from build123d import *

# Parameters (mm, degrees)
SKETCH_R        = 1.2
PAD_DEPTH       = 7
SKETCH001_W     = 3.3
SKETCH001_H     = 5
POCKET_DEPTH    = 50
SKETCH002_W     = 3.3
SKETCH002_H     = 5
POCKET001_DEPTH = 30
CHAMFER_SIZE    = 2.5
FILLET_R        = 1
FILLET001_R     = 1


with BuildPart() as part:
    # Sketch → Pad (new body)
    with BuildSketch(Plane.XY):
        Polygon((-4.5, 23), (4.5, 23), (4.5, 4.5), (9.5, 4.5), (9.5, -4.5), (4.5, -4.5), (4.5, -23), (-4.5, -23), (-4.5, -4.5), (-9.5, -4.5), (-9.5, 4.5), (-4.5, 4.5), align=None)
        with Locations((0, 15.5)):
            Circle(SKETCH_R, mode=Mode.SUBTRACT)
        with Locations((0, -15.5)):
            Circle(SKETCH_R, mode=Mode.SUBTRACT)
    extrude(amount=PAD_DEPTH)

    # Sketch001 → Pocket (cut)
    with BuildSketch(Plane(origin=(0, 23, 0), x_dir=(-1, 0, 0), z_dir=(0, 1, 0))):
        with Locations((0, 4.5)):
            Rectangle(SKETCH001_W, SKETCH001_H)
    extrude(amount=-POCKET_DEPTH, mode=Mode.SUBTRACT)

    # Sketch002 → Pocket001 (cut)
    with BuildSketch(Plane(origin=(-9.5, 0, 0), x_dir=(0, -1, 0), z_dir=(-1, 0, 0))):
        with Locations((0, 4.5)):
            Rectangle(SKETCH002_W, SKETCH002_H)
    extrude(amount=-POCKET001_DEPTH, mode=Mode.SUBTRACT)

    # Chamfer
    chamfer_edges = [part.edges().sort_by_distance(p)[0] for p in [
        (-4.5, 13.75, 7),
        (-7, 4.5, 7),
        (4.5, 13.75, 7),
        (7, 4.5, 7),
        (7, -4.5, 7),
        (4.5, -13.75, 7),
        (-4.5, -13.75, 7),
        (-7, -4.5, 7),
    ]]
    chamfer(chamfer_edges, length=CHAMFER_SIZE)

    # Fillet
    fillet_edges = [part.edges().sort_by_distance(p)[0] for p in [
        (-9.5, 1.65, 4.5),
        (-9.5, -1.65, 4.5),
        (-1.65, 23, 4.5),
        (1.65, 23, 4.5),
        (9.5, 1.65, 4.5),
        (9.5, -1.65, 4.5),
        (-1.65, -23, 4.5),
        (1.65, -23, 4.5),
        (1.65, 1.65, 4.5),
        (-1.65, 1.65, 4.5),
        (1.65, -1.65, 4.5),
        (-1.65, -1.65, 4.5),
    ]]
    fillet(fillet_edges, radius=FILLET_R)

    # Fillet001
    fillet001_edges = [part.edges().sort_by_distance(p)[0] for p in [
        (-9.5, -4.5, 2.25),
        (-9.5, 4.5, 2.25),
        (-4.5, 4.5, 2.25),
        (-4.5, 23, 2.25),
        (4.5, 23, 2.25),
        (4.5, 4.5, 2.25),
        (9.5, 4.5, 2.25),
        (9.5, -4.5, 2.25),
        (4.5, -4.5, 2.25),
        (4.5, -23, 2.25),
        (-4.5, -23, 2.25),
        (-4.5, -4.5, 2.25),
    ]]
    fillet(fillet001_edges, radius=FILLET001_R)


solid = part.part
Can you work these out from the model? Positions are in its coordinate system, mm. A direction names the side the tool comes from. Give positions to 0.01 mm unless a question says otherwise; leave off trailing zeros. Loops run counter-clockwise (first coordinate to the right, second up) from the corner with the lowest first, then second, coordinate; pieces in that order, holes last. Notation, with made-up numbers: (49, 65) -> (56, 65) arc R22 cw to (56, 103) -> close; hole circle Ø9 at (74, -31.5). An arc over 180 degrees is marked (long way). Write item = value, one per line.
1) Suppose I cut it at C-C on x = -4. Write out the boundary of the cut face in (y, z), then the cut area to 3 significant figures.
Check result:
outline = (-22.87, 0) -> (22.87, 0) -> (22.87, 5) -> (4, 5) -> (2, 7) -> (1.65, 7) -> (1.65, 2) -> (-1.65, 2) -> (-1.65, 7) -> (-2, 7) -> (-4, 5) -> (-22.87, 5) -> close
area = 224 mm2
2) Thinking about a two-plate mould opening in Y: for faces 1 (the flat face through (-9.5, 0, 1.7)), 2 (the cylindrical face through (-9.215, 4.199, 2.177)), 3 (the cylindrical face through (-9.215, 1.951, 4.535)), which applies, released by +Y, released by -Y, zero draft, split by the parting line, or undercut?
Check result:
face_1 = zero draft
face_2 = released by +Y
face_3 = undercut
3) Suppose I cut it at A-A on y = 15.5. Write out the boundary of the cut face in (x, z).
Check result:
outline = (-4.5, 0) -> (-1.2, 0) -> (-1.2, 2) -> (-1.65, 2) -> (-1.65, 7) -> (-2, 7) -> (-4.5, 4.5) -> close; (1.2, 0) -> (4.5, 0) -> (4.5, 4.5) -> (2, 7) -> (1.65, 7) -> (1.65, 2) -> (1.2, 2) -> close
4) Suppose I cut it at B-B on x = 7.75. Write out the boundary of the cut face in (y, z).
Check result:
outline = (-4.5, 0) -> (4.5, 0) -> (4.5, 4.5) -> (2, 7) -> (1.65, 7) -> (1.65, 2) -> (-1.65, 2) -> (-1.65, 7) -> (-2, 7) -> (-4.5, 4.5) -> close
5) Will these pins go through, and if not, where does the flat tip stop? pin 1 (1.5 mm diameter, centred on x = -4.5, z = 5, fed in from +Y); pin 2 (3 mm diameter, centred on x = 6.5, z = 4.5, fed in from -Y); pin 3 (3.5 mm diameter, centred on y = -12, z = 1.5, fed in from -X).
Check result:
pin_1 = 22.97
pin_2 = -4.63
pin_3 = -4.5
6) I need wall thicknesses on L1, parallel to Y at x = 0, z = 0.4; L2, parallel to X at y = -15.5, z = 0.75; L3, parallel to X at y = -17.5, z = 3. Which ranges of each line are inside material? Lowest first, please. Write a range as from..to.
Check result:
L1 = -23..-16.7, -14.3..14.3, 16.7..23
L2 = -4.5..-1.2, 1.2..4.5
L3 = -4.5..-1.65, 1.65..4.5
7) For faces 4 (the flat face through (7, 4.5, 2)), 5 (the flat face through (-7, -4.5, 2)), 6 (the flat face through (-7, -3, 6)), 7 (the flat face through (-7, 4.5, 2)), which set-ups out of +Z, -Z, +X, -X, +Y, -Y let a thin tool reach every point of the face, with its end or its side?
Check result:
face_4 = +Z, -Z, +X, +Y
face_5 = +Z, -Z, -X, -Y
face_6 = +Z, -X, -Y
face_7 = +Z, -Z, -X, +Y
